Design review of the part built by this model. Coordinates are the model's own, in mm. A direction names the side the tool comes from. Coordinates: 2 decimals unless noted, no trailing zeros. Order: outer loops, then holes, each group sorted by start corner. A loop starts at its lowest first (then second) coordinate and runs counter-clockwise, first axis right, second up. Notation, with made-up numbers: M -33,-23.5 L -14,-23.5 A11 ccw -14,-5.5 Z; hole C 19.5,54.25 d3. An arc over 180 degrees is marked long. Answer in a Markdown table with one row per item.
from build123d import *

# Parameters (mm, degrees)
CYLINDER059_R              = 1.5
CYLINDER059_DEPTH          = 45
CYLINDER060_R              = 1.5
CYLINDER060_DEPTH          = 45
PRISM006_DEPTH             = 3
PRISM007_DEPTH             = 3
CYLINDER061_R              = 3
CYLINDER061_DEPTH          = 5
CYLINDER043_R              = 4
CYLINDER043_DEPTH          = 40
CYLINDER045_R              = 7
CYLINDER045_DEPTH          = 2
CYLINDER044_R              = 7
CYLINDER044_DEPTH          = 2
EXTRUDE010_DEPTH           = 12
EXTRUDE023_DEPTH           = 24
CYLINDER046_R              = 1.6
CYLINDER046_DEPTH          = 10
CYLINDER062_R              = 3
CYLINDER062_DEPTH          = 5
BOX012_W                   = 31
BOX012_H                   = 60
BOX012_DEPTH               = 6
BOX011_W                   = 61
BOX011_H                   = 60
BOX011_DEPTH               = 6
EXTRUDE015_DEPTH           = 6
EXTRUDE015_PLACEMENT_ANGLE = 90
EXTRUDE011_DEPTH           = 10
EXTRUDE024_DEPTH           = 10
EXTRUDE009_DEPTH           = 18


with BuildPart() as cilindro059:
    # Cylinder059 → Cylinder059 (new body)
    with BuildSketch(Plane(origin=(98, -36, -87), x_dir=(0, 0, 1), z_dir=(-1, 0, 0))):
        Circle(CYLINDER059_R)
    extrude(amount=CYLINDER059_DEPTH)


with BuildPart() as cilindro060:
    # Cylinder060 → Cylinder060 (new body)
    with BuildSketch(Plane(origin=(98, 36, -87), x_dir=(0, 0, 1), z_dir=(-1, 0, 0))):
        Circle(CYLINDER060_R)
    extrude(amount=CYLINDER060_DEPTH)


with BuildPart() as prisma006:
    # Prism006 → Prism006 (new body)
    with BuildSketch(Plane(origin=(65, -36, -87), x_dir=(0, 0, 1), z_dir=(-1, 0, 0))):
        Polygon((3, 0), (1.5, 2.598076), (-1.5, 2.598076), (-3, 0), (-1.5, -2.598076), (1.5, -2.598076), align=None)
    extrude(amount=PRISM006_DEPTH)


with BuildPart() as prisma007:
    # Prism007 → Prism007 (new body)
    with BuildSketch(Plane(origin=(65, 36, -87), x_dir=(0, 0, 1), z_dir=(-1, 0, 0))):
        Polygon((3, 0), (1.5, 2.598076), (-1.5, 2.598076), (-3, 0), (-1.5, -2.598076), (1.5, -2.598076), align=None)
    extrude(amount=PRISM007_DEPTH)


with BuildPart() as cilindro061:
    # Cylinder061 → Cylinder061 (new body)
    with BuildSketch(Plane(origin=(89, -36, -87), x_dir=(0, 0, 1), z_dir=(-1, 0, 0))):
        Circle(CYLINDER061_R)
    extrude(amount=CYLINDER061_DEPTH)


with BuildPart() as cilindro043:
    # Cylinder043 → Cylinder043 (new body)
    with BuildSketch(Plane(origin=(83, -20, 55), x_dir=(1, 0, 0), z_dir=(0, 1, 0))):
        Circle(CYLINDER043_R)
    extrude(amount=CYLINDER043_DEPTH)


with BuildPart() as cilindro045:
    # Cylinder045 → Cylinder045 (new body)
    with BuildSketch(Plane(origin=(83, 10, 55), x_dir=(1, 0, 0), z_dir=(0, 1, 0))):
        Circle(CYLINDER045_R)
    extrude(amount=CYLINDER045_DEPTH)


with BuildPart() as fusion020:
    # Cylinder044 → Cylinder044 (new body)
    with BuildSketch(Plane(origin=(83, -12, 55), x_dir=(1, 0, 0), z_dir=(0, 1, 0))):
        Circle(CYLINDER044_R)
    extrude(amount=CYLINDER044_DEPTH)

    # Fusion020: union Cilindro045
    add(cilindro045.part)


with BuildPart() as cut012:
    # Sketch010 → Extrude010 (new body, symmetric)
    with BuildSketch(Plane.XZ):
        with BuildLine():
            ThreePointArc((77.817442, 35.68314), (89.140517, 35.965977), (98.494144, 42.353597))
            Line((98.494144, 42.353597), (108, 54))
            Line((108, 54), (108, 85))
            Line((58, 85), (108, 85))
            Line((58, 41), (58, 85))
            Line((77.817442, 35.68314), (58, 41))
        make_face()
    extrude(amount=EXTRUDE010_DEPTH, both=True)

    # Cut012: cut Fusion020
    add(fusion020.part, mode=Mode.SUBTRACT)


with BuildPart() as extrude023:
    # Sketch015 → Extrude023 (new body)
    with BuildSketch(Plane.XY.offset(-75)):
        with BuildLine():
            Line((-74, 21), (-74, -21))
            ThreePointArc((-74, -21), (-67.384986, -70.729267), (-48, -117))
            Line((-48, -117), (48, -117))
            ThreePointArc((48, -117), (67.384986, -70.729267), (74, -21))
            Line((74, 21), (74, -21))
            ThreePointArc((74, 21), (67.384986, 70.729267), (48, 117))
            Line((-48, 117), (48, 117))
            ThreePointArc((-48, 117), (-67.384986, 70.729267), (-74, 21))
        make_face()
    extrude(amount=-EXTRUDE023_DEPTH)


with BuildPart() as cono:
    # Cone → Cone (revolve)
    with BuildSketch(Plane(origin=(0, 0, -96), x_dir=(1, 0, 0), z_dir=(0, -1, 0))):
        Polygon((0, 0), (1.6, 0), (4.1, 3), (0, 3), align=None)
    revolve(axis=Axis((0, 0, -96), (0, 0, 1)))


with BuildPart() as cilindro046:
    # Cylinder046 → Cylinder046 (new body)
    with BuildSketch(Plane.XY.offset(-106)):
        Circle(CYLINDER046_R)
    extrude(amount=CYLINDER046_DEPTH)


with BuildPart() as fusion029:
    # Fusion029 base: copy of Cilindro046
    add(cilindro046.part)

    # Fusion029: union Cono
    add(cono.part)


with BuildPart() as fusion029_1:
    # Fusion029 placement: moved
    add(fusion029.part.moved(Location((128, -27, 0))))


with BuildPart() as fusion028:
    # Fusion028 base: copy of Cilindro046
    add(cilindro046.part)

    # Fusion028: union Cono
    add(cono.part)


with BuildPart() as fusion028_1:
    # Fusion028 placement: moved
    add(fusion028.part.moved(Location((116, 68, 0))))


with BuildPart() as fusion052:
    # Cylinder062 → Cylinder062 (new body)
    with BuildSketch(Plane(origin=(89, 36, -87), x_dir=(0, 0, 1), z_dir=(-1, 0, 0))):
        Circle(CYLINDER062_R)
    extrude(amount=CYLINDER062_DEPTH)

    # Fusion052: union Cilindro059, Cilindro060, Prisma006, Prisma007, Cilindro061, Cilindro043, Cut012, Extrude023, Fusion029, Fusion028
    add(cilindro059.part)
    add(cilindro060.part)
    add(prisma006.part)
    add(prisma007.part)
    add(cilindro061.part)
    add(cilindro043.part)
    add(cut012.part)
    add(extrude023.part)
    add(fusion029_1.part)
    add(fusion028_1.part)


with BuildPart() as cubo011:
    # Box012 → Box012 (new body)
    with BuildSketch(Plane(origin=(65, -78, -99), x_dir=(1, 0, 0), z_dir=(0, 0, 1))):
        with Locations((15.5, 30)):
            Rectangle(BOX012_W, BOX012_H)
    extrude(amount=BOX012_DEPTH)


with BuildPart() as cubo010:
    # Box011 → Box011 (new body)
    with BuildSketch(Plane(origin=(65, 18, -99), x_dir=(1, 0, 0), z_dir=(0, 0, 1))):
        with Locations((30.5, 30)):
            Rectangle(BOX011_W, BOX011_H)
    extrude(amount=BOX011_DEPTH)


with BuildPart() as fusion024:
    # Sketch012 → Extrude015 (new body)
    with BuildSketch(Plane.XY.offset(-99)):
        with BuildLine():
            ThreePointArc((0, 10), (-10, 0), (0, -10))
            Line((20, -10), (0, -10))
            Line((20, 10), (20, -10))
            Line((0, 10), (20, 10))
        make_face()
    extrude(amount=EXTRUDE015_DEPTH)


with BuildPart() as fusion024_1:
    # Extrude015 placement: moved
    add(fusion024.part.moved(Location((128, -27, 0))).rotate(Axis((128, -27, 0), (0, 0, 1)), EXTRUDE015_PLACEMENT_ANGLE))

    # Fusion024: union Cubo011, Cubo010
    add(cubo011.part)
    add(cubo010.part)


with BuildPart() as extrude011:
    # Sketch011 → Extrude011 (new body)
    with BuildSketch(Plane.YZ.offset(78)):
        Polygon((-70.523409, -93), (-18, -93), (-18, 37), align=None)
        Polygon((18, -93), (18, 37), (70.523409, -93), align=None)
    extrude(amount=EXTRUDE011_DEPTH)


with BuildPart() as extrude024:
    # Sketch016 → Extrude024 (new body)
    with BuildSketch(Plane.YZ.offset(70)):
        Polygon((-40, -78), (-60, -93), (60, -93), (40, -78), align=None)
    extrude(amount=EXTRUDE024_DEPTH)


with BuildPart() as soporte_eje:
    # Sketch009 → Extrude009 (new body, symmetric)
    with BuildSketch(Plane.XZ):
        with BuildLine():
            Line((74, -99), (74, 29.524522))
            ThreePointArc((74, 29.524522), (72.771088, 35.470709), (69.285714, 40.442584))
            ThreePointArc((102.212801, 49.444079), (77.725993, 74.292093), (69.285714, 40.442584))
            Line((102.212801, 49.444079), (97.329592, 32.557567))
            ThreePointArc((97.329592, 32.557567), (98.526548, -32.428153), (136.199214, -85.393678))
            Line((154, -99), (136.199214, -85.393678))
            Line((74, -99), (154, -99))
        make_face()
    extrude(amount=EXTRUDE009_DEPTH, both=True)

    # Fusion053: union Fusion024, Extrude011, Extrude024
    add(fusion024_1.part)
    add(extrude011.part)
    add(extrude024.part)

    # Cut020: cut Fusion052
    add(fusion052.part, mode=Mode.SUBTRACT)


solid = soporte_eje.part
(1) For line 1 along Y through (x, z) = (128, -97.6); line 2 along X through (y, z) = (-27, -97.3); line 3 along Z through (x, y) = (83, -15.5), list the stretches that pass through material, from the lowest coordinate up. Write a range as from..to.
Return value:
| item | result |
|---|---|
| line 1 | y = -37..-28.6, -25.4..18 |
| line 2 | x = 73.91..96, 118..126.4, 129.6..138 |
| line 3 | z = -99..51, 59..75 |
(2) Add section C-C, the plane z = -10. Give the boundary of the cut face in (x, y).
Return value:
| item | result |
|---|---|
| outline | M 74,-18 L 78,-18 L 78,-36.99 L 88,-36.99 L 88,-18 L 93.66,-18 L 93.66,18 L 88,18 L 88,36.99 L 78,36.99 L 78,18 L 74,18 Z |
(3) Add section D-D, the plane y = -66. Give the boundary of the cut face in (x, z).
Return value:
| item | result |
|---|---|
| outline | M 68.6,-99 L 96,-99 L 96,-93 L 88,-93 L 88,-81.8 L 78,-81.8 L 78,-93 L 68.6,-93 Z |
(4) Insertion check: pin 1 Ø20 at (x, z) = (91, 49.5) entering from -Y; pin 2 Ø5 at (y, z) = (-36, -87) entering from +X; pin 3 Ø21 at (x, y) = (124, -24) entering from +Z; pin 4 Ø2.5 at (y, z) = (36, -87) entering from -X. Each pin has a flat end and moves straight along its axis. Give the tip position at first contact, or say it passes through.
Return value:
| item | result |
|---|---|
| pin 1 | stops at y = -18 |
| pin 2 | stops at x = 84 |
| pin 3 | stops at z = -64.51 |
| pin 4 | passes through |
(5) For faces 5 (the flat face through (78, -33, -42)), 6 (the flat face through (86, -10, 58)), 7 (the flat face through (74, 0, -34)), 8 (the flat face through (99.26, -0.25, 39.24)), 9 (the flat face through (83, 12, 46)), list the 3-axis set-ups (+Z, -Z, +X, -X, +Y, -Y) from which the entire face can be reached by the end or side of a thin tool; tool diameter is ignored.
Return value:
| item | result |
|---|---|
| face 5 | +Z, -X, -Y |
| face 6 | +Z, +X, -X |
| face 7 | -Z, -X |
| face 8 | +X, +Y, -Y |
| face 9 | none |
(6) Add section A-A, the plane z = 55. Give the boundary of the cut face in (x, y), and give its area (3 significant figures).
Return value:
| item | result |
|---|---|
| outline | M 63,-18 L 79,-18 L 79,-10 L 76,-10 L 76,-12 L 63,-12 Z; M 63,12 L 76,12 L 76,10 L 79,10 L 79,18 L 63,18 Z; M 87,-18 L 103,-18 L 103,-12 L 90,-12 L 90,-10 L 87,-10 Z; M 87,10 L 90,10 L 90,12 L 103,12 L 103,18 L 87,18 Z |
| area | 408 mm2 |
(7) Draft analysis for pull direction X (two halves, no side actions). For faces 1 (the cylindrical face through (72.717, 43.058, -90.686)), 2 (the conical face through (114.606, 66.931, -95.812)), 3 (the flat face through (88, -33, -56)), 4 (the cylindrical face through (82.133, -14.056, 58.905)), state which applies: pulls with the +X half, pulls with the -X half, needs draft (parallel to the pull), parting line crosses it, or undercut.
Return value:
| item | result |
|---|---|
| face 1 | pulls with the -X half |
| face 2 | undercut |
| face 3 | pulls with the +X half |
| face 4 | undercut |
(8) Add section B-B, the plane y = -42.5. Give the boundary of the cut face in (x, z) (3 decimals), and give its area (3 significant figures).
Return value:
| item | result |
|---|---|
| outline | M 72.781,-99 L 96,-99 L 96,-93 L 88,-93 L 88,-23.64 L 78,-23.64 L 78,-79.875 L 72.781,-79.875 Z |
| area | 901 mm2 |
